from build123d import *

# Parameters (mm, degrees)
F0_W           = 30
F0_H           = 60
F1_DEPTH       = 8
F2_D           = 5.5
F2_DEPTH       = 30
F2_CBORE_D     = 9
F2_CBORE_DEPTH = 5.5
F2_TIP         = 1.6523667023
F3_W           = 4
F3_H           = 2.5
F4_DEPTH       = 30.001


with BuildPart() as f1:
    # F0 (on Top) → F1 (new body)
    with BuildSketch(Plane.XY):
        Rectangle(F0_W, F0_H)
    extrude(amount=F1_DEPTH)

    # F2
    with Locations(Plane(origin=(0, 0, 0), x_dir=(1, 0, 0), z_dir=(0, 0, -1))):
        with Locations((0, 8)):
            CounterBoreHole(F2_D / 2, F2_CBORE_D / 2, F2_CBORE_DEPTH, depth=F2_DEPTH)
            with Locations((0, 0, -(F2_DEPTH + F2_TIP / 2))):  # 118° drill point
                Cone(0, F2_D / 2, F2_TIP, mode=Mode.SUBTRACT)

    # F3 (on face) → F4 (cut, through all)
    with BuildSketch(Plane(origin=(-15, 0, 0), x_dir=(0, -1, 0), z_dir=(-1, 0, 0))):
        with Locations((-19.8, 4)):
            Rectangle(F3_W, F3_H)
        with Locations((0, 4)):
            Rectangle(F3_W, F3_H)
        with Locations((19.8, 4)):
            Rectangle(F3_W, F3_H)
    extrude(amount=-F4_DEPTH, mode=Mode.SUBTRACT)


solid = f1.part
For this review, take the finished solid that the model builds, in its own axes (mm). A direction names the side the tool comes from. Give positions to 0.01 mm unless a question says otherwise; leave off trailing zeros. Loops run counter-clockwise (first coordinate to the right, second up) from the corner with the lowest first, then second, coordinate; pieces in that order, holes last.
Item 1: Insertion check: pin 1 (14.5 mm diameter, centred on x = 0, y = -8, fed in from +Z). The pin has a flat end and moves straight along its axis. Give the tip position at first contact, or say it passes through.
Item 2: Take a section at C-C, the plane z = 4.25. State the section outline as (x, y) points, and give its area (3 significant figures).
Item 3: Take a section at D-D, the plane x = -12.25. State the section outline as (y, z) points.
Item 4: Take a section at B-B, the plane x = 0. State the section outline as (y, z) points, and give its area (3 significant figures).
Item 5: Take a section at A-A, the plane y = 19.5. State the section outline as (x, z) points, and give its area (3 significant figures).
Item 6: For line 1 along Y through (x, z) = (4.75, 3.5); line 2 along Y through (x, z) = (0, 6.65); line 3 along Z through (x, y) = (3, 21.5), list the stretches that pass through material, from the lowest coordinate up.
Item 7: Tool access review of faces 4 (the flat face through (0, 0, 8)), 5 (the flat face through (0, 0, 5.25)), 6 (the flat face through (0, -5, 5.5)): name each direction out of +Z, -Z, +X, -X, +Y, -Y from which nothing blocks a thin tool from reaching the whole face with its end or side.
Item 8: Draft analysis for pull direction Y (two halves, no side actions). For faces 1 (the flat face through (0, 21.8, 4)), 2 (the flat face through (0, 30, 4)), 3 (the flat face through (-15, 0, 6)), state which applies: +Y half, -Y half, draft (parallel to the pull), parting line (faces both ways), or undercut.
Calculated:
1. pin 1: stops at z = 8
2. outline: (-15, -30) - (15, -30) - (15, -21.8) - (-15, -21.8) - close; (-15, -17.8) - (15, -17.8) - (15, -2) - (-15, -2) - close; (-15, 2) - (15, 2) - (15, 17.8) - (-15, 17.8) - close; (-15, 21.8) - (15, 21.8) - (15, 30) - (-15, 30) - close; hole circle Ø9 at (0, -8)
2. area: 1,380 mm2
3. outline: (-30, 0) - (30, 0) - (30, 8) - (-30, 8) - close; hole (-21.8, 2.75) - (-17.8, 2.75) - (-17.8, 5.25) - (-21.8, 5.25) - close; hole (-2, 2.75) - (2, 2.75) - (2, 5.25) - (-2, 5.25) - close; hole (17.8, 2.75) - (21.8, 2.75) - (21.8, 5.25) - (17.8, 5.25) - close
4. outline: (-30, 0) - (-12.5, 0) - (-12.5, 5.5) - (-10.75, 5.5) - (-10.75, 8) - (-30, 8) - close; (-5.25, 5.5) - (-3.5, 5.5) - (-3.5, 0) - (30, 0) - (30, 8) - (-5.25, 8) - close; hole (-21.8, 2.75) - (-17.8, 2.75) - (-17.8, 5.25) - (-21.8, 5.25) - close; hole (-2, 2.75) - (2, 2.75) - (2, 5.25) - (-2, 5.25) - close; hole (17.8, 2.75) - (21.8, 2.75) - (21.8, 5.25) - (17.8, 5.25) - close
4. area: 387 mm2
5. outline: (-15, 0) - (15, 0) - (15, 2.75) - (-15, 2.75) - close; (-15, 5.25) - (15, 5.25) - (15, 8) - (-15, 8) - close
5. area: 165 mm2
6. line 1: y = -30 to -21.8, -17.8 to -2, 2 to 17.8, 21.8 to 30
6. line 2: y = -30 to -10.75, -5.25 to 30
6. line 3: z = 0 to 2.75, 5.25 to 8
7. face 4: +Z, +X, -X, +Y, -Y
7. face 5: +X, -X
7. face 6: -Z
8. face 1: undercut
8. face 2: +Y half
8. face 3: draft
